Autodesk Inventor part; units mm, degrees
ref_plane "YZ Plane" through (0, 0, 0) normal (1, 0, 0) x (0, 1, 0)
ref_plane "XZ Plane" through (0, 0, 0) normal (0, 1, 0) x (-1, 0, 0)
ref_plane "XY Plane" through (0, 0, 0) normal (0, 0, 1) x (1, 0, 0)
sketch "Sketch1" plane through (0, 0, 0) normal (0, 1, 0) x (-1, 0, 0)
  circle A0 centre (0, 0) radius 5
  dimension "d0" = 10
extrude "Extrusion1" add sketch "Sketch1" along normal blind 15
sketch "Sketch2" plane through (0, 15, 0) normal (0, 1, 0) x (1, 0, 0)
  circle A0 centre (0, 0) radius 2.65
  dimension "d3" = 5.3
extrude "Extrusion2" cut sketch "Sketch2" against normal blind 8
sketch "Sketch3" plane through (0, 0, 0) normal (0, -1, 0) x (1, 0, 0)
  line L0 (-1.6271, -1.2616) -> (1.6271, -1.2616)
  line L1 (1.6271, -1.2616) -> (1.6271, 1.2616)
  line L2 (1.6271, 1.2616) -> (-1.6271, 1.2616)
  line L3 (-1.6271, 1.2616) -> (-1.6271, -1.2616)
  circle A0 centre (0, 0) radius 5
  line L4 (-1.6271, -1.2616) -> (1.6271, 1.2616) construction
  line L5 (1.6271, -1.2616) -> (-1.6271, 1.2616) construction
extrude "Extrusion3" add sketch "Sketch3" along normal blind 5 contours L3 L2 L1 L0
sketch "Sketch4" plane through (-1.6271, 0, 1.2616) normal (0, 0, 1) x (1, 0, 0)
  circle A0 centre (1.6271, -14.7217) radius 13.1898
  arc A1 (5.8054, -5.9844) -> (10.354, -10.5216) centre (1.6271, -14.7217) ccw
  line L0 (1.6271, -14.7217) -> (13.5121, -9.0018)
  line L1 (1.6271, -14.7217) -> (7.5696, -2.2953)
  point P0 (1.6271, 0)
  point P1 (13.8416, -19.6992)
  point P2 (11.3121, -5.7679)
  point P3 (10.354, -10.5216)
  point P4 (7.3175, -2.8225)
extrude "Extrusion4" add sketch "Sketch4" against normal blind 2.512 contours A0 L1 A1 L0
sketch "Sketch5" plane through (0, 15, 0) normal (0, 1, 0) x (1, 0, 0)
  line L0 (-4, 1.6583) -> (-0.5639, 4.2933)
  line L1 (-0.5639, 4.2933) -> (3.4361, 2.6349)
  line L2 (3.4361, 2.6349) -> (4, -1.6583)
  line L3 (4, -1.6583) -> (0.5639, -4.2933)
  line L4 (0.5639, -4.2933) -> (-3.4361, -2.6349)
  line L5 (-3.4361, -2.6349) -> (-4, 1.6583)
  point P0 (0, 0)
  point P1 (0, 0)
  point P2 (-1.4361, -3.4641)
  dimension "d10" = 8
  dimension "d11" = 7.5
extrude "Extrusion5" cut sketch "Sketch5" against normal blind 1
properties part number "OriginNutipt" material "Thermoplastic Resin"
CAD build for the part. Positions are in the model's coordinates, mm. A direction names the side the tool comes from. Give positions to 0.01 mm unless a question says otherwise; leave off trailing zeros. Write each loop counter-clockwise with the first axis right and the second up, starting at its lowest first coordinate (ties: lowest second). Pieces come first, ordered by that corner, then holes. Notation, with made-up numbers: M 65.5,2 L 78.5,2 A16 ccw 78.5,12 Z; hole C 47,-2 d9. An arc over 180 degrees is marked long. Put each result on its own line as item: value. Start each with the question number.
(1) Band-saw the part on B-B, the plane y = -20.5. Write the cut outline in (x, z), and give its area (3 significant figures).
(2) Mould opens along Z. For faces 6 (the face through (3.714, 14.507, -0.518)), 7 (the face through (-7.103, -21.305, 0.023)), 8 (the face through (1.08, 7.4, 4.88)) say: +Z half, -Z half, draft (parallel to the pull), parting line (faces both ways), or undercut.
(3) Probe L1, parallel to X at y = -15, z = 0.25; L2, parallel to Y at x = 3.25, z = -0.5; L3, parallel to Y at x = -3.5, z = -2.5. List the from-to ranges inside material, lowest first.
(4) Flat gauge pins, fed straight in: pin 1 Ø5 at (x, z) = (7.5, 1.5) entering from +Y; pin 2 Ø1 at (y, z) = (10, -3.5) entering from -X; pin 3 Ø4 at (x, z) = (0, -0.5) entering from +Y. Where does each tip first touch, or does it go through?
(5) Band-saw the part on C-C, the plane z = 0.5. Write the cut outline in (x, y) (3 decimals), and give its area (3 significant figures).
(6) Band-saw the part on D-D, the plane y = 11.5. Write the cut outline in (x, z), and give its area (3 significant figures).
(7) Which spindle directions (+Z, -Z, +X, -X, +Y, -Y) get a long thin tool onto all of the face, cutting with end or side? Do faces 1 (the face through (-3, -24.2, 1.262)), 2 (the face through (-2, 0, 0)), 3 (the face through (-3.714, 14.507, 0.518)), 4 (the face through (10.284, -9.772, 0.023)), 5 (the face through (0, -2, -1.262)). Say none if no direction does.
Response values:
1. outline: M -11.86,-1.25 L -7.77,-1.25 L -7.77,1.26 L -11.86,1.26 Z; M 7.77,-1.25 L 11.86,-1.25 L 11.86,1.26 L 7.77,1.26 Z
1. area: 20.5 mm2
2. face 6: undercut
2. face 7: draft
2. face 8: parting line
3. L1: x = -13.19 to -9.68, 9.68 to 13.19
3. L2: y = -27.5 to -23.85, -5.6 to -1.94, 0 to 14
3. L3: y = 0 to 15
4. pin 1: stops at y = -2.52
4. pin 2: stops at x = -4
4. pin 3: stops at y = 7
5. outline: M -4.975,0 L -1.627,0 L -1.627,-1.633 A13.19 ccw long 11.885,-9.002 L 8.727,-10.522 A9.685 cw long 4.178,-5.984 L 5.69,-2.823 A13.19 ccw 1.627,-1.633 L 1.627,0 L 4.975,0 L 4.975,15 L 3.848,15 L 3.848,14 L 2.602,14 L 2.602,7 L -2.602,7 L -2.602,14 L -3.717,14 L -3.717,15 L -4.975,15 Z
5. area: 335 mm2
6. outline: C 0,0 d10; hole C 0,0 d5.3
6. area: 56.5 mm2
7. face 1: +Z, +X, -X, -Y
7. face 2: none
7. face 3: +Y
7. face 4: +Z, -Z, +Y
7. face 5: -Z, +X, -X, -Y
